Could you check a few things on this model? Use its own coordinates, in mm. Face numbers are marked on the shaded views. A direction names the side the tool comes from. Round coordinates to 2 decimals unless told otherwise and drop trailing zeros. Order: outer loops, then holes, each group sorted by start corner. A loop starts at its lowest first (then second) coordinate and runs counter-clockwise, first axis right, second up. Notation, with made-up numbers: (50, 32.25) -> (67, 32.25) arc R18 ccw to (67, 51.25) -> close; hole circle Ø5 at (51.5, 4). An arc over 180 degrees is marked (long way). One line per question, with ' | ' between items.
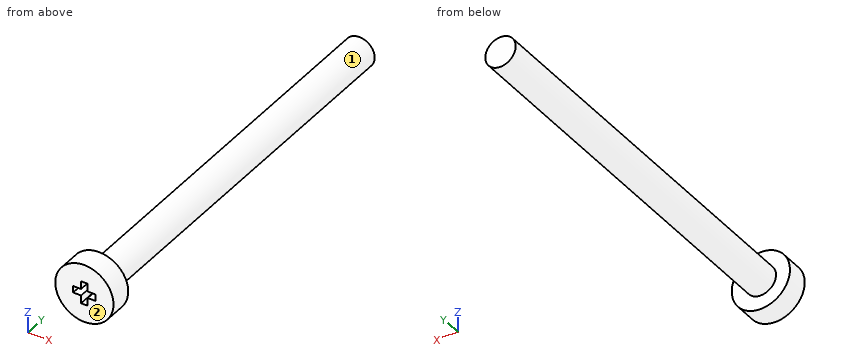
```python
from build123d import *

# Parameters (mm, degrees)
SKETCH_1_R          = 2.2
EXTRUDE_1_DEPTH     = 1.7
EXTRUDE_START       = 1.7
SKETCH_1_4_R        = 1.15
EXTRUDE_2_DEPTH     = 30
SKETCH_1_3_W        = 1.7
SKETCH_1_3_H        = 0.5
SKETCH_1_3_W_2      = 0.5
SKETCH_1_3_H_2      = 1.7
CUT_EXTRUDE_1_DEPTH = 1.5


with BuildPart() as part:
    # 草图1 → 凸台-拉伸1 (new body)
    with BuildSketch(Plane(origin=(0, 0, 0), x_dir=(1, 0, 0), z_dir=(0, 1, 0))):
        with Locations(Location((0, 0, 0), (0, 0, 270))):
            Circle(SKETCH_1_R)
    extrude(amount=EXTRUDE_1_DEPTH)

    # 草图1<4> → 凸台-拉伸2 (add)
    with BuildSketch(Plane(origin=(0, 0, 0), x_dir=(1, 0, 0), z_dir=(0, 1, 0)).offset(EXTRUDE_START)):
        with Locations(Location((0, 0, 0), (0, 0, 270))):
            Circle(SKETCH_1_4_R)
    extrude(amount=EXTRUDE_2_DEPTH)

    # 草图1<3> → 切除-拉伸1 (cut)
    with BuildSketch(Plane(origin=(0, 0, 0), x_dir=(1, 0, 0), z_dir=(0, 1, 0))):
        Rectangle(SKETCH_1_3_W, SKETCH_1_3_H)
        Rectangle(SKETCH_1_3_W_2, SKETCH_1_3_H_2)
    extrude(amount=CUT_EXTRUDE_1_DEPTH, mode=Mode.SUBTRACT)


solid = part.part
```
1. I want a section at B-B on y = 27. List the corners of the cut face in (x, z) for me, and give its area (3 significant figures).
From the geometry:
outline: circle Ø2.3 at (0, 0) | area: 4.15 mm²
2. I want a section at A-A on x = 0.55. List the corners of the cut face in (y, z) for me.
From the geometry:
outline: (0, -2.13) -> (1.7, -2.13) -> (1.7, -1.01) -> (31.7, -1.01) -> (31.7, 1.01) -> (1.7, 1.01) -> (1.7, 2.13) -> (0, 2.13) -> (0, 0.25) -> (1.5, 0.25) -> (1.5, -0.25) -> (0, -0.25) -> close
3. I want a section at D-D on x = 1.8. List the corners of the cut face in (y, z) for me, and give its area (3 significant figures).
From the geometry:
outline: (0, -1.26) -> (1.7, -1.26) -> (1.7, 1.26) -> (0, 1.26) -> close | area: 4.30 mm²
4. On a 3-axis mill with a long thin cutter (end or side, diameter ignored), from which of +Z, -Z, +X, -X, +Y, -Y can I reach the whole of each face in a straight line? I mean the marked faces 1 and 2. Say none if no direction works.
From the geometry:
face 1: +Y | face 2: +Z, -Z, +X, -X, -Y
5. I'm going to push flat-ended pins straight in: pin 1 (0.7 mm diameter, centred on x = -0.5, y = 1, fed in from +Z); pin 2 (0.7 mm diameter, centred on x = 0.5, y = 1, fed in from -Z); pin 3 (1.5 mm diameter, centred on y = 8, z = -1, fed in from +X). Where does each tip first touch, or does it pass through?
From the geometry:
pin 1: stops at z = 2.19 | pin 2: stops at z = -2.19 | pin 3: stops at x = 1.12
6. I want a section at C-C on z = 1.75. List the corners of the cut face in (x, y) for me.
From the geometry:
outline: (-1.33, 0) -> (1.33, 0) -> (1.33, 1.7) -> (-1.33, 1.7) -> close
7. I need wall thicknesses on probe 1 along Y at (x, z) = (0.1, 1.65); probe 2 along Z at (x, y) = (0.1, 19); probe 3 along X at (y, z) = (29.5, 0.9). Which ranges of each line are inside material? Lowest first, please.
From the geometry:
probe 1: y = 0 to 1.7 | probe 2: z = -1.15 to 1.15 | probe 3: x = -0.72 to 0.72
